Autodesk Inventor part; units mm, degrees
ref_plane "YZ Plane" through (0, 0, 0) normal (1, 0, 0) x (0, 1, 0)
ref_plane "XZ Plane" through (0, 0, 0) normal (0, 1, 0) x (-1, 0, 0)
ref_plane "XY Plane" through (0, 0, 0) normal (0, 0, 1) x (1, 0, 0)
sketch "Sketch1" plane through (0, 0, 0) normal (0, 0, 1) x (1, 0, 0)
  line L0 (3.9408, -0.7944) -> (3.5592, -0.7944)
  line L1 (1.4408, -0.7944) -> (1.0592, -0.7944)
  line L2 (-1.0592, -0.7944) -> (-1.4408, -0.7944)
  line L3 (-3.5592, -0.7944) -> (-3.9408, -0.7944)
  line L4 (-6.0592, -0.7944) -> (-6.25, -0.7944)
  line L5 (6.25, -0.7944) -> (6.0592, -0.7944)
  line L6 (6.25, -0.7944) -> (6.25, -8.7944)
  line L7 (6.25, -8.7944) -> (-6.25, -8.7944)
  line L8 (-6.25, -8.7944) -> (-6.25, -0.7944)
  line L9 (-6.25, -0.7944) -> (-6.0592, -0.7944)
  line L10 (-3.9408, -0.7944) -> (-3.5592, -0.7944)
  line L11 (-1.4408, -0.7944) -> (-1.0592, -0.7944)
  line L12 (1.0592, -0.7944) -> (1.4408, -0.7944)
  line L13 (3.5592, -0.7944) -> (3.9408, -0.7944)
  line L14 (6.0592, -0.7944) -> (6.25, -0.7944)
  line L15 (-6.25, -0.7944) -> (6.25, -0.7944)
  point P0 (0, 0)
  dimension "height" = 8
extrude "Extrusion1" add sketch "Sketch1" against normal blind 15
hole "Hole1" at (-0.125, -8.7944, -2.5) direction (0, 1, 0) diameter 2.459 end through all
hole "Hole2" at (6.25, -4.7944, -7.5) direction (-1, 0, 0) diameter 3.242 end through all
equation "\"d12\" = 0.5 * width"
equation "\"d13\" = 0.5 * height"
properties part number "T2.5 belt holder" material "Aluminum 6061"
Read the model definition and answer for the solid it produces. Units are mm, in the model's axes. Give positions to 0.01 mm unless a question says otherwise; leave off trailing zeros. Loops run counter-clockwise (first coordinate to the right, second up) from the corner with the lowest first, then second, coordinate; pieces in that order, holes last.
Item 1: This flat-tipped pin is pushed along its axis until it touches: pin 1 Ø2 at (y, z) = (-3.5, -7) entering from -X. Where does it stop, or does it pass through?
Item 2: The part is cut by section D-D (x = 4.5). Write down the section's boundary in (y, z).
Item 3: Find the intervals of material crossed by line 1 along X through (y, z) = (-4, -2.5); line 2 along Y through (x, z) = (-1.5, -7.5); line 3 along Z through (x, y) = (0, -6), in increasing order.
Item 4: The part is cut by section B-B (y = -6). Give the number of separate pieces and of enclosed holes in the cut face, and give its area (3 significant figures).
Item 5: The mould has two halves that part along X. Classify faces 1 (the flat face through (0, -5, -15)), 2 (the flat face through (6.25, -4.7, -5.7)), 3 (the cylindrical face through (-0.494, -4.738, -3.673)), 4 (the flat face through (-6.25, -4.9, -5.7)): released by +X, released by -X, zero draft, split by the parting line, or undercut.
Item 6: The part is cut by section C-C (z = -7.5). Write down the section's boundary in (x, y), and give its area (3 significant figures).
Item 7: The part is cut by section A-A (z = -2.5). Write down the section's boundary in (x, y), and give its area (3 significant figures).
Taken from the geometry:
1. pin 1: stops at x = -6.25
2. outline: (-8.79, -15) - (-0.79, -15) - (-0.79, 0) - (-8.79, 0) - close; hole circle Ø3.24 at (-4.79, -7.5)
3. line 1: x = -6.25 to -1.35, 1.1 to 6.25
3. line 2: y = -8.79 to -6.42, -3.17 to -0.79
3. line 3: z = -15 to -8.58, -6.42 to -3.72, -1.28 to 0
4. separate pieces: 2
4. enclosed holes: 1
4. area: 156 mm2
5. face 1: zero draft
5. face 2: released by +X
5. face 3: undercut
5. face 4: released by -X
6. outline: (-6.25, -8.79) - (6.25, -8.79) - (6.25, -6.42) - (-6.25, -6.42) - close; (-6.25, -3.17) - (6.25, -3.17) - (6.25, -0.79) - (-6.25, -0.79) - close
6. area: 59.5 mm2
7. outline: (-6.25, -8.79) - (-1.35, -8.79) - (-1.35, -0.79) - (-6.25, -0.79) - close; (1.1, -8.79) - (6.25, -8.79) - (6.25, -0.79) - (1.1, -0.79) - close
7. area: 80.3 mm2
